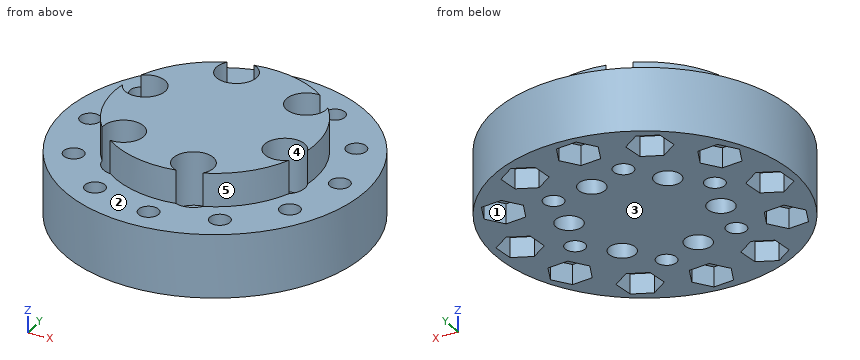
```python
from build123d import *

# Parameters (mm, degrees)
SKETCH_1_R               = 22.5
EXTRUDE_1_DEPTH          = 9.5
SKETCH_2_R               = 15
EXTRUDE_2_DEPTH          = 5
SKETCH_3_R               = 1.5
CUT_EXTRUDE_1_DEPTH      = 5
SKETCH_5_R               = 1.5
CUT_EXTRUDE_2_DEPTH      = 34.207679835
CUT_EXTRUDE_6_DEPTH      = 3
PATTERN_CIRCULAR_1_COUNT = 12
SKETCH_6_R               = 1.5
CUT_EXTRUDE_3_DEPTH      = 35.96784237
SKETCH_7_R               = 3
CUT_EXTRUDE_4_DEPTH      = 8
PATTERN_CIRCULAR_2_COUNT = 6
SKETCH_8_R               = 2
CUT_EXTRUDE_5_DEPTH      = 4
PATTERN_CIRCULAR_3_COUNT = 6


with BuildPart() as part:
    # 草图1 → 凸台-拉伸1 (new body)
    with BuildSketch(Plane.XY):
        Circle(SKETCH_1_R)
    extrude(amount=EXTRUDE_1_DEPTH)

    # 草图2 → 凸台-拉伸2 (add)
    with BuildSketch(Plane.XY.offset(9.5)):
        Circle(SKETCH_2_R)
    extrude(amount=EXTRUDE_2_DEPTH)

    # 草图3 → 切除-拉伸1 (cut)
    with BuildSketch(Plane.XY.offset(9.5)):
        with Locations((0, 18.5)):
            Circle(SKETCH_3_R)
    cut_extrude_1 = extrude(amount=-CUT_EXTRUDE_1_DEPTH, mode=Mode.SUBTRACT)

    # 草图5 → 切除-拉伸2 (cut, through all)
    with BuildSketch(Plane.XY.offset(9.5)):
        with Locations((0, 18.5)):
            Circle(SKETCH_5_R)
    cut_extrude_2 = extrude(amount=-CUT_EXTRUDE_2_DEPTH, mode=Mode.SUBTRACT)

    # 草图9 → 切除-拉伸6 (cut)
    with BuildSketch(Plane(origin=(0, 0, 0), x_dir=(-1, 0, 0), z_dir=(0, 0, -1))):
        Polygon((1.204492644, 21.438116881), (-1.942237536, 21.012179669), (-3.14673018, 18.074062788), (-1.204492644, 15.561883119), (1.942237536, 15.987820331), (3.14673018, 18.925937212), align=None)
    cut_extrude_6 = extrude(amount=-CUT_EXTRUDE_6_DEPTH, mode=Mode.SUBTRACT)

    # 阵列(圆周)1: 切除-拉伸1, 切除-拉伸2, 切除-拉伸6 ×12 about axis
    pattern_circular_1_axis = Axis((0, 0, 0), (0, 0, 1))
    add([cut_extrude_1.rotate(pattern_circular_1_axis, i * 360 / PATTERN_CIRCULAR_1_COUNT) for i in range(1, PATTERN_CIRCULAR_1_COUNT)], mode=Mode.SUBTRACT)
    add([cut_extrude_2.rotate(pattern_circular_1_axis, i * 360 / PATTERN_CIRCULAR_1_COUNT) for i in range(1, PATTERN_CIRCULAR_1_COUNT)], mode=Mode.SUBTRACT)
    add([cut_extrude_6.rotate(pattern_circular_1_axis, i * 360 / PATTERN_CIRCULAR_1_COUNT) for i in range(1, PATTERN_CIRCULAR_1_COUNT)], mode=Mode.SUBTRACT)

    # 草图6 → 切除-拉伸3 (cut, through all)
    with BuildSketch(Plane(origin=(0, 0, 0), x_dir=(-1, 0, 0), z_dir=(0, 0, -1))):
        with Locations((3.235238064, 12.074072829)):
            Circle(SKETCH_6_R)
    cut_extrude_3 = extrude(amount=-CUT_EXTRUDE_3_DEPTH, mode=Mode.SUBTRACT)

    # 草图7 → 切除-拉伸4 (cut)
    with BuildSketch(Plane.XY.offset(14.5)):
        with Locations((-3.235238064, 12.074072829)):
            Circle(SKETCH_7_R)
    cut_extrude_4 = extrude(amount=-CUT_EXTRUDE_4_DEPTH, mode=Mode.SUBTRACT)

    # 阵列(圆周)2: 切除-拉伸3, 切除-拉伸4 ×6 about axis
    pattern_circular_2_axis = Axis((0, 0, 0), (0, 0, 1))
    add([cut_extrude_3.rotate(pattern_circular_2_axis, i * 360 / PATTERN_CIRCULAR_2_COUNT) for i in range(1, PATTERN_CIRCULAR_2_COUNT)], mode=Mode.SUBTRACT)
    add([cut_extrude_4.rotate(pattern_circular_2_axis, i * 360 / PATTERN_CIRCULAR_2_COUNT) for i in range(1, PATTERN_CIRCULAR_2_COUNT)], mode=Mode.SUBTRACT)

    # 草图8 → 切除-拉伸5 (cut)
    with BuildSketch(Plane(origin=(0, 0, 0), x_dir=(-1, 0, 0), z_dir=(0, 0, -1))):
        with Locations((-2.63995426, 9.852443428)):
            Circle(SKETCH_8_R)
    cut_extrude_5 = extrude(amount=-CUT_EXTRUDE_5_DEPTH, mode=Mode.SUBTRACT)

    # 阵列(圆周)3: 切除-拉伸5 ×6 about axis
    pattern_circular_3_axis = Axis((0, 0, 0), (0, 0, 1))
    for i in range(1, PATTERN_CIRCULAR_3_COUNT):
        add(cut_extrude_5.rotate(pattern_circular_3_axis, i * 360 / PATTERN_CIRCULAR_3_COUNT), mode=Mode.SUBTRACT)


solid = part.part
```
The listing builds one solid part. Answer for the finished solid, in the listing's coordinates (mm). Face numbers are marked on the shaded views. A direction names the side the tool comes from. Give positions to 0.01 mm unless a question says otherwise; leave off trailing zeros. Order: outer loops, then holes, each group sorted by start corner. A loop starts at its lowest first (then second) coordinate and runs counter-clockwise, first axis right, second up. Notation, with made-up numbers: (39.5, -2.5) - (95.5, -2.5) arc R24 ccw to (95.5, 9.5) - close; hole circle Ø3 at (4, -29.5). An arc over 180 degrees is marked (long way). Use one line per item in the form item = value. Start each with the question number.
(1) A cutting plane is placed at A-A, the plane x = 4. Write down the section's boundary in (y, z), then the cut area to 3 significant figures.
(2) Consider line 1 (X direction, y = 10, z = 8.25) (1 decimal); line 2 (Y direction, x = 0, z = 5.5); line 3 (Y direction, x = -11, z = 8.5). Determine where each line is inside the solid, lowest interval first. Write a range as from..to.
(3) The mould has two halves that part along Y. Classify the marked faces 3, 4 and 5: released by +Y, released by -Y, zero draft, split by the parting line, or undercut.
(4) A cutting plane is placed at B-B, the plane z = 12.75. Write down the section's boundary in (x, y).
(5) For the marked faces 1 and 2, determine the directions among +Z, -Z, +X, -X, +Y, -Y from which every point of the face is accessible in a straight line to the end or side of a thin tool.
(6) Flat-ended cylindrical pins translate along their axes: pin 1 Ø1.8 at (x, y) = (17, -1) entering from -Z; pin 2 Ø2.5 at (x, y) = (-7.21, 7.21) entering from -Z; pin 3 Ø1.5 at (x, z) = (15.5, 7.5) entering from -Y. Find the tip coordinate at first contact, or state that the pin passes through.
Ans:
q1.outline = (-22.14, 0) - (-13.36, 0) - (-13.36, 6.5) - (-14.97, 6.5) - (-14.97, 9.5) - (-22.14, 9.5) - close; (-10.78, 0) - (8.39, 0) - (8.39, 4) - (11.32, 4) - (11.32, 0) - (22.14, 0) - (22.14, 9.5) - (14.46, 9.5) - (14.46, 14.5) - (-9.17, 14.5) - (-9.17, 6.5) - (-10.78, 6.5) - close
q1.area = 493 mm^2
q2.line_1 = -20.2..-17.3, -14.7..-5.4, -1.1..6.1, 11.6..14.7, 17.3..20.2
q2.line_2 = -22.5..-20, -17..17, 20..22.5
q2.line_3 = -19.63..-10.92, -6.76..0.43, 6.04..19.63
q3.face_3 = zero draft
q3.face_4 = undercut
q3.face_5 = released by -Y
q4.outline = (-14.85, 2.1) arc R15 ccw to (-11.81, -9.25) arc R3 cw (long way) to (-9.25, -11.81) arc R15 ccw to (2.1, -14.85) arc R3 cw (long way) to (5.61, -13.91) arc R15 ccw to (13.91, -5.61) arc R3 cw (long way) to (14.85, -2.1) arc R15 ccw to (11.81, 9.25) arc R3 cw (long way) to (9.25, 11.81) arc R15 ccw to (-2.1, 14.85) arc R3 cw (long way) to (-5.61, 13.91) arc R15 ccw to (-13.91, 5.61) arc R3 cw (long way) to start
q5.face_1 = -Z
q5.face_2 = +Z
q6.pin_1 = 3
q6.pin_2 = 4
q6.pin_3 = -16.99
